Part model, mm, in its own coordinate system. A direction names the side the tool comes from. Give positions to 0.01 mm unless a question says otherwise; leave off trailing zeros. Order: outer loops, then holes, each group sorted by start corner. A loop starts at its lowest first (then second) coordinate and runs counter-clockwise, first axis right, second up.
from build123d import *

# Parameters (mm, degrees)
BOX010_W                = 22
BOX010_H                = 10
BOX010_DEPTH            = 10
BOX010_ROLL_ANGLE       = 45
BOX009_W                = 22
BOX009_H                = 10
BOX009_DEPTH            = 10
BOX009_ROLL_ANGLE       = 45
CYLINDER010_R           = 1.5
CYLINDER010_DEPTH       = 40
CYLINDER010_PITCH_ANGLE = 90
CYLINDER011_R           = 1.5
CYLINDER011_DEPTH       = 40
CYLINDER011_PITCH_ANGLE = 90
CYLINDER012_R           = 1.5
CYLINDER012_DEPTH       = 40
CYLINDER012_PITCH_ANGLE = 90
CYLINDER009_R           = 1.5
CYLINDER009_DEPTH       = 40
CYLINDER009_PITCH_ANGLE = 90
BOX004_W                = 2
BOX004_H                = 32
BOX004_DEPTH            = 6
CYLINDER_R              = 11.2
CYLINDER_DEPTH          = 25
CYLINDER001_R           = 13.5
CYLINDER001_DEPTH       = 18
CYLINDER001_PITCH_ANGLE = 90
CYLINDER003_R           = 1.4
CYLINDER003_DEPTH       = 20
CYLINDER003_PITCH_ANGLE = 90
CYLINDER005_R           = 1.4
CYLINDER005_DEPTH       = 20
CYLINDER005_PITCH_ANGLE = 90
CYLINDER004_R           = 1.4
CYLINDER004_DEPTH       = 20
CYLINDER004_PITCH_ANGLE = 90
CYLINDER002_R           = 1.4
CYLINDER002_DEPTH       = 20
CYLINDER002_PITCH_ANGLE = 90
BOX002_W                = 6
BOX002_H                = 7
BOX002_DEPTH            = 20
BOX006_W                = 4.5
BOX006_H                = 7
BOX006_DEPTH            = 16
BOX007_W                = 4.5
BOX007_H                = 7
BOX007_DEPTH            = 16
BOX008_W                = 4.5
BOX008_H                = 7
BOX008_DEPTH            = 16
BOX005_W                = 4.5
BOX005_H                = 7
BOX005_DEPTH            = 16
BOX003_W                = 6
BOX003_H                = 7
BOX003_DEPTH            = 20
BOX001_W                = 6
BOX001_H                = 32
BOX001_DEPTH            = 30
BOX_W                   = 24
BOX_H                   = 32
BOX_DEPTH               = 25
FILLET_R                = 4
FILLET001_R             = 4
FILLET002_R             = 4
FILLET003_R             = 4


with BuildPart() as cube010:
    # Box010 → Box010 (new body)
    with BuildSketch(Plane.XY):
        with Locations((11, 5)):
            Rectangle(BOX010_W, BOX010_H)
    extrude(amount=BOX010_DEPTH)


with BuildPart() as cube010_1:
    # Box010 roll: moved
    add(cube010.part.rotate(Axis((0, 0, 0), (1, 0, 0)), BOX010_ROLL_ANGLE))


with BuildPart() as cube010_2:
    # Box010 placement: moved
    add(cube010_1.part.moved(Location((2, 41, -7))))


with BuildPart() as fusionwingcuts:
    # Box009 → Box009 (new body)
    with BuildSketch(Plane.XY):
        with Locations((11, 5)):
            Rectangle(BOX009_W, BOX009_H)
    extrude(amount=BOX009_DEPTH)


with BuildPart() as fusionwingcuts_1:
    # Box009 roll: moved
    add(fusionwingcuts.part.rotate(Axis((0, 0, 0), (1, 0, 0)), BOX009_ROLL_ANGLE))


with BuildPart() as fusionwingcuts_2:
    # Box009 placement: moved
    add(fusionwingcuts_1.part.moved(Location((2, -9, -7))))

    # Fusion005: union Cube010
    add(cube010_2.part)


with BuildPart() as fusionwingcuts_3:
    # Fusion005 placement: moved
    add(fusionwingcuts_2.part.moved(Location((0, 0, 5.5))))


with BuildPart() as cylinder010:
    # Cylinder010 → Cylinder010 (new body)
    with BuildSketch(Plane.XY):
        Circle(CYLINDER010_R)
    extrude(amount=CYLINDER010_DEPTH)


with BuildPart() as cylinder010_1:
    # Cylinder010 pitch: moved
    add(cylinder010.part.rotate(Axis((0, 0, 0), (0, 1, 0)), CYLINDER010_PITCH_ANGLE))


with BuildPart() as cylinder010_2:
    # Cylinder010 placement: moved
    add(cylinder010_1.part.moved(Location((0, -3.5, 6))))


with BuildPart() as cylinder011:
    # Cylinder011 → Cylinder011 (new body)
    with BuildSketch(Plane.XY):
        Circle(CYLINDER011_R)
    extrude(amount=CYLINDER011_DEPTH)


with BuildPart() as cylinder011_1:
    # Cylinder011 pitch: moved
    add(cylinder011.part.rotate(Axis((0, 0, 0), (0, 1, 0)), CYLINDER011_PITCH_ANGLE))


with BuildPart() as cylinder011_2:
    # Cylinder011 placement: moved
    add(cylinder011_1.part.moved(Location((0, 35.5, 12))))


with BuildPart() as cylinder012:
    # Cylinder012 → Cylinder012 (new body)
    with BuildSketch(Plane.XY):
        Circle(CYLINDER012_R)
    extrude(amount=CYLINDER012_DEPTH)


with BuildPart() as cylinder012_1:
    # Cylinder012 pitch: moved
    add(cylinder012.part.rotate(Axis((0, 0, 0), (0, 1, 0)), CYLINDER012_PITCH_ANGLE))


with BuildPart() as cylinder012_2:
    # Cylinder012 placement: moved
    add(cylinder012_1.part.moved(Location((0, 35.5, 6))))


with BuildPart() as fusionwingscrews:
    # Cylinder009 → Cylinder009 (new body)
    with BuildSketch(Plane.XY):
        Circle(CYLINDER009_R)
    extrude(amount=CYLINDER009_DEPTH)


with BuildPart() as fusionwingscrews_1:
    # Cylinder009 pitch: moved
    add(fusionwingscrews.part.rotate(Axis((0, 0, 0), (0, 1, 0)), CYLINDER009_PITCH_ANGLE))


with BuildPart() as fusionwingscrews_2:
    # Cylinder009 placement: moved
    add(fusionwingscrews_1.part.moved(Location((0, -3.5, 12))))

    # Fusion004: union Cylinder010, Cylinder011, Cylinder012
    add(cylinder010_2.part)
    add(cylinder011_2.part)
    add(cylinder012_2.part)


with BuildPart() as fusionwingscrews_3:
    # Fusion004 placement: moved
    add(fusionwingscrews_2.part.moved(Location((0, 0, 5.5))))


with BuildPart() as obj1:
    # Box004 → Box004 (new body)
    with BuildSketch(Plane(origin=(-4, 0, 10), x_dir=(1, 0, 0), z_dir=(0, 0, 1))):
        with Locations((1, 16)):
            Rectangle(BOX004_W, BOX004_H)
    extrude(amount=BOX004_DEPTH)


with BuildPart() as cylinderheatsink:
    # Cylinder → Cylinder (new body)
    with BuildSketch(Plane(origin=(6.4, 16, 0), x_dir=(1, 0, 0), z_dir=(0, 0, 1))):
        Circle(CYLINDER_R)
    extrude(amount=CYLINDER_DEPTH)


with BuildPart() as cylinderfan:
    # Cylinder001 → Cylinder001 (new body)
    with BuildSketch(Plane.XY):
        Circle(CYLINDER001_R)
    extrude(amount=CYLINDER001_DEPTH)


with BuildPart() as cylinderfan_1:
    # Cylinder001 pitch: moved
    add(cylinderfan.part.rotate(Axis((0, 0, 0), (0, 1, 0)), CYLINDER001_PITCH_ANGLE))


with BuildPart() as cylinderfan_2:
    # Cylinder001 placement: moved
    add(cylinderfan_1.part.moved(Location((13, 16, 15))))


with BuildPart() as obj2:
    # Cylinder003 → Cylinder003 (new body)
    with BuildSketch(Plane.XY):
        Circle(CYLINDER003_R)
    extrude(amount=CYLINDER003_DEPTH)


with BuildPart() as obj2_1:
    # Cylinder003 pitch: moved
    add(obj2.part.rotate(Axis((0, 0, 0), (0, 1, 0)), CYLINDER003_PITCH_ANGLE))


with BuildPart() as obj2_2:
    # Cylinder003 placement: moved
    add(obj2_1.part.moved(Location((20, 4, 27))))


with BuildPart() as obj3:
    # Cylinder005 → Cylinder005 (new body)
    with BuildSketch(Plane.XY):
        Circle(CYLINDER005_R)
    extrude(amount=CYLINDER005_DEPTH)


with BuildPart() as obj3_1:
    # Cylinder005 pitch: moved
    add(obj3.part.rotate(Axis((0, 0, 0), (0, 1, 0)), CYLINDER005_PITCH_ANGLE))


with BuildPart() as obj3_2:
    # Cylinder005 placement: moved
    add(obj3_1.part.moved(Location((20, 28, 3))))


with BuildPart() as obj4:
    # Cylinder004 → Cylinder004 (new body)
    with BuildSketch(Plane.XY):
        Circle(CYLINDER004_R)
    extrude(amount=CYLINDER004_DEPTH)


with BuildPart() as obj4_1:
    # Cylinder004 pitch: moved
    add(obj4.part.rotate(Axis((0, 0, 0), (0, 1, 0)), CYLINDER004_PITCH_ANGLE))


with BuildPart() as obj4_2:
    # Cylinder004 placement: moved
    add(obj4_1.part.moved(Location((20, 28, 27))))


with BuildPart() as fusioncuts:
    # Cylinder002 → Cylinder002 (new body)
    with BuildSketch(Plane.XY):
        Circle(CYLINDER002_R)
    extrude(amount=CYLINDER002_DEPTH)


with BuildPart() as fusioncuts_1:
    # Cylinder002 pitch: moved
    add(fusioncuts.part.rotate(Axis((0, 0, 0), (0, 1, 0)), CYLINDER002_PITCH_ANGLE))


with BuildPart() as fusioncuts_2:
    # Cylinder002 placement: moved
    add(fusioncuts_1.part.moved(Location((20, 4, 3))))

    # Fusion001: union obj2, obj3, obj4
    add(obj2_2.part)
    add(obj3_2.part)
    add(obj4_2.part)

    # Fusion: union FusionWingCuts, FusionWingScrews, obj1, CylinderHeatSink, CylinderFan
    add(fusionwingcuts_3.part)
    add(fusionwingscrews_3.part)
    add(obj1.part)
    add(cylinderheatsink.part)
    add(cylinderfan_2.part)


with BuildPart() as obj5:
    # Box002 → Box002 (new body)
    with BuildSketch(Plane(origin=(-6, 0, 0), x_dir=(1, 0, 0), z_dir=(0, 0, 1))):
        with Locations((3, 3.5)):
            Rectangle(BOX002_W, BOX002_H)
    extrude(amount=BOX002_DEPTH)


with BuildPart() as cube006:
    # Box006 → Box006 (new body)
    with BuildSketch(Plane(origin=(19, -7, 0), x_dir=(1, 0, 0), z_dir=(0, 0, 1))):
        with Locations((2.25, 3.5)):
            Rectangle(BOX006_W, BOX006_H)
    extrude(amount=BOX006_DEPTH)


with BuildPart() as cube007:
    # Box007 → Box007 (new body)
    with BuildSketch(Plane(origin=(2, 32, 0), x_dir=(1, 0, 0), z_dir=(0, 0, 1))):
        with Locations((2.25, 3.5)):
            Rectangle(BOX007_W, BOX007_H)
    extrude(amount=BOX007_DEPTH)


with BuildPart() as cube008:
    # Box008 → Box008 (new body)
    with BuildSketch(Plane(origin=(19, 32, 0), x_dir=(1, 0, 0), z_dir=(0, 0, 1))):
        with Locations((2.25, 3.5)):
            Rectangle(BOX008_W, BOX008_H)
    extrude(amount=BOX008_DEPTH)


with BuildPart() as fusionwings:
    # Box005 → Box005 (new body)
    with BuildSketch(Plane(origin=(2, -7, 0), x_dir=(1, 0, 0), z_dir=(0, 0, 1))):
        with Locations((2.25, 3.5)):
            Rectangle(BOX005_W, BOX005_H)
    extrude(amount=BOX005_DEPTH)

    # Fusion006: union Cube006, Cube007, Cube008
    add(cube006.part)
    add(cube007.part)
    add(cube008.part)


with BuildPart() as fusionwings_1:
    # Fusion006 placement: moved
    add(fusionwings.part.moved(Location((0, 0, 5.5))))


with BuildPart() as obj6:
    # Box003 → Box003 (new body)
    with BuildSketch(Plane(origin=(-6, 25, 0), x_dir=(1, 0, 0), z_dir=(0, 0, 1))):
        with Locations((3, 3.5)):
            Rectangle(BOX003_W, BOX003_H)
    extrude(amount=BOX003_DEPTH)


with BuildPart() as obj7:
    # Box001 → Box001 (new body)
    with BuildSketch(Plane(origin=(24, 0, 0), x_dir=(1, 0, 0), z_dir=(0, 0, 1))):
        with Locations((3, 16)):
            Rectangle(BOX001_W, BOX001_H)
    extrude(amount=BOX001_DEPTH)


with BuildPart() as obj8:
    # Box → Box (new body)
    with BuildSketch(Plane.XY):
        with Locations((12, 16)):
            Rectangle(BOX_W, BOX_H)
    extrude(amount=BOX_DEPTH)

    # Fusion007: union obj5, FusionWings, obj6, obj7
    add(obj5.part)
    add(fusionwings_1.part)
    add(obj6.part)
    add(obj7.part)

    # Fillet
    fillet_edges = [obj8.edges().sort_by_distance(p)[0] for p in [
        (-6, 3.5, 0),
    ]]
    fillet(fillet_edges, radius=FILLET_R)

    # Fillet001
    fillet001_edges = [obj8.edges().sort_by_distance(p)[0] for p in [
        (12, 0, 0),
    ]]
    fillet(fillet001_edges, radius=FILLET001_R)

    # Fillet002
    fillet002_edges = [obj8.edges().sort_by_distance(p)[0] for p in [
        (12, 32, 0),
    ]]
    fillet(fillet002_edges, radius=FILLET002_R)

    # Fillet003
    fillet003_edges = [obj8.edges().sort_by_distance(p)[0] for p in [
        (-6, 26.5, 0),
    ]]
    fillet(fillet003_edges, radius=FILLET003_R)

    # Cut: cut FusionCUTS
    add(fusioncuts_2.part, mode=Mode.SUBTRACT)


solid = obj8.part
Item 1: Band-saw the part on B-B on y = -3.5. List the corners of the cut face in (x, z).
Item 2: Band-saw the part on C-C on z = 3. List the corners of the cut face in (x, y), plus the area to 3 significant figures.
Item 3: Drill centre lines: probe 1 along X at (y, z) = (-2.5, 13.5); probe 2 along Y at (x, z) = (-2, 19); probe 3 along Y at (x, z) = (3, 17). Where is each one in solid material? Low to high.
Item 4: Band-saw the part on A-A on x = -1. List the corners of the cut face in (y, z), plus the area to 3 significant figures.
Item 5: Band-saw the part on D-D on y = 17. List the corners of the cut face in (x, z), plus the area to 3 significant figures.
Item 6: Which spindle directions (+Z, -Z, +X, -X, +Y, -Y) get a long thin tool onto all of the face, cutting with end or side? Do faces 4 (the face through (21, 33, 5.5)), 5 (the face through (2, -3.5, 13.4)), 6 (the face through (6.5, -3.5, 13.4)), 7 (the face through (-3, 29, 10)). Say none if no direction does.
Item 7: Pull direction Y, two halves, no side cores. Call faces 1 (the face through (-1.9, 25, 9.86)), 2 (the face through (21.22, -4.43, 8.07)), 3 (the face through (-3, 4, 16)): released by +Y, released by -Y, zero draft, split by the parting line, or undercut.
Item 8: Drop flat-ended pins along their axis: P1, Ø2, axis at y = -2, z = 10, coming from the +X side; P2, Ø12, axis at x = 11, y = 16, coming from the -Z side; P3, Ø3.5, axis at y = 36, z = 14.5, coming from the -X side; P4, Ø2, axis at x = 15.5, y = 2, coming from the +Z side. Give the stop position or say it passes through.
Working result:
1. outline: (2, 7.14) - (6.5, 7.14) - (6.5, 10) - (2, 10) - close; (2, 13) - (6.5, 13) - (6.5, 16) - (2, 16) - close; (2, 19) - (6.5, 19) - (6.5, 21.5) - (2, 21.5) - close; (19, 7.14) - (23.5, 7.14) - (23.5, 10) - (19, 10) - close; (19, 13) - (23.5, 13) - (23.5, 16) - (19, 16) - close; (19, 19) - (23.5, 19) - (23.5, 21.5) - (19, 21.5) - close
2. outline: (-5.87, 4) arc R3.87 ccw to (-2, 0.13) - (30, 0.13) - (30, 2.6) - (20, 2.6) - (20, 5.4) - (30, 5.4) - (30, 9.82) - (15.74, 9.82) arc R11.2 cw to (-0.27, 7) - (-5.87, 7) - close; (-5.87, 25) - (-0.27, 25) arc R11.2 cw to (15.74, 22.18) - (30, 22.18) - (30, 26.6) - (20, 26.6) - (20, 29.4) - (30, 29.4) - (30, 31.87) - (-2, 31.87) arc R3.87 ccw to (-5.87, 28) - close
2. area: 478 mm2
3. probe 1: x = 2 to 6.5, 19 to 23.5
3. probe 2: y = 0 to 7, 25 to 32
3. probe 3: y = -7 to -4.91, -2.09 to 5.33, 26.67 to 34.09, 36.91 to 39
4. outline: (0, 4) arc R4 ccw to (4, 0) - (7, 0) - (7, 20) - (0, 20) - close; (25, 0) - (28, 0) arc R4 ccw to (32, 4) - (32, 20) - (25, 20) - close
4. area: 273 mm2
5. outline: (17.56, 0) - (30, 0) - (30, 1.54) - (17.56, 1.54) - close; (24, 28.46) - (30, 28.46) - (30, 30) - (24, 30) - close
5. area: 28.4 mm2
6. face 4: -Z, +X, -X, +Y
6. face 5: +Z, -Z, -X, -Y
6. face 6: +Z, -Z, -Y
6. face 7: +Y, -Y
7. face 1: undercut
7. face 2: released by -Y
7. face 3: zero draft
8. P1: stops at x = 23.5
8. P2: passes through
8. P3: stops at x = 2
8. P4: stops at z = 25
